Input: dimensioned drawing with shaded views. Units: mm. Origin: part minimum x, y, z. Give positions to 0.01 mm unless a question says otherwise; leave off trailing zeros. Write each loop counter-clockwise with the first axis right and the second up, starting at its lowest first coordinate (ties: lowest second). Pieces come first, ordered by that corner, then holes.
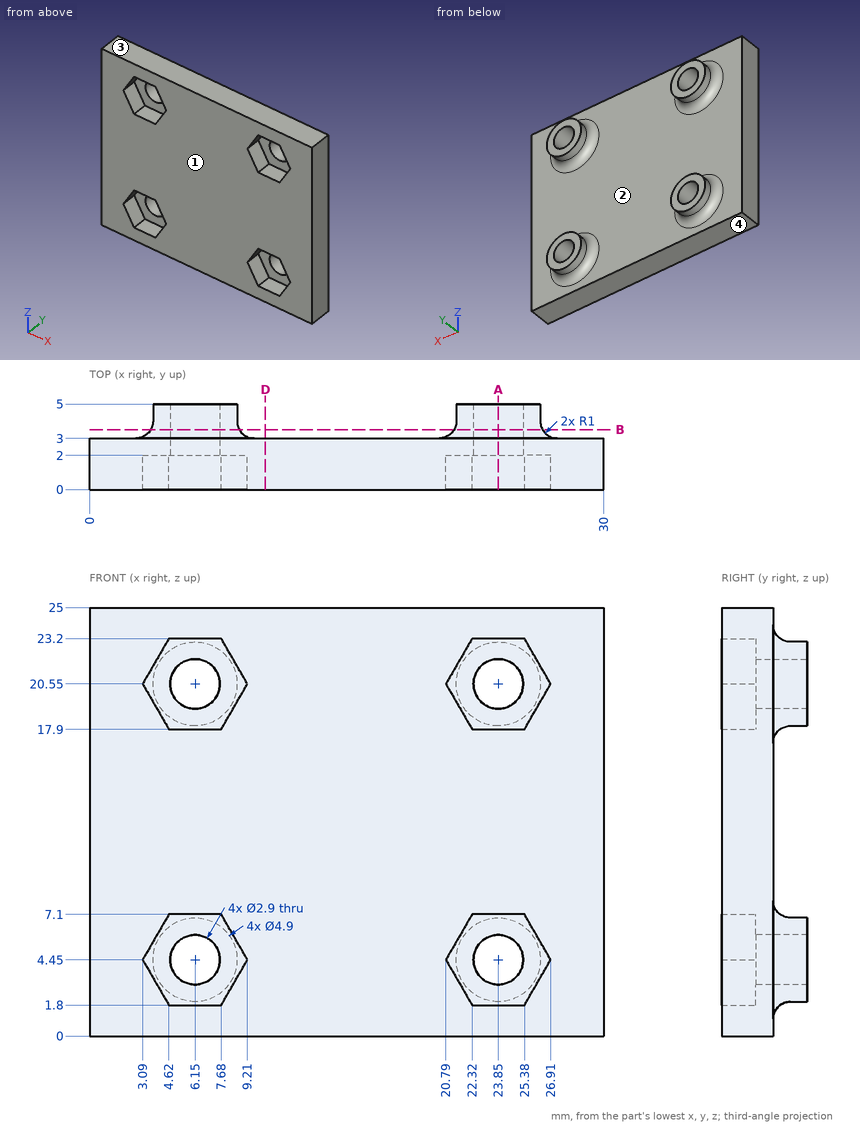
Item 1: Section B-B (y = 3.5). Return loops of the section in (x, z), and give its area (3 significant figures).
Item 2: Mould query, pull axis Z, two halves, no side actions, for the marked faces 1, 2, 3 and 4. Classes: +Z half, -Z half, draft (parallel to the pull), parting line (faces both ways), or undercut.
Item 3: Section D-D (x = 10.25). Return loops of the section in (y, z), and give its area (3 significant figures).
Item 4: Ray query, line 1 (Z direction, x = 6, y = 1.55); line 2 (Z direction, x = 6.15, y = 2.6); line 3 (X direction, y = 3.55, z = 4.45). Return the intervals inside material, ascending.
Item 5: Pin query (flat end, axial travel): pin 1 (1.6 mm diameter, centred on x = 23, z = 21.5, fed in from -Y); pin 2 (12 mm diameter, centred on x = 15, z = 5.5, fed in from +Y). Return the tip coordinate at first contact, or that it passes through.
Item 6: Section A-A (x = 23.85). Give the number of separate pieces and of enclosed holes in the cut face, and give its area (3 significant figures).
Solved:
1. outline: circle Ø5.17 at (6.15, 4.45); circle Ø5.17 at (6.15, 20.55); circle Ø5.17 at (23.85, 4.45); circle Ø5.17 at (23.85, 20.55); hole circle Ø2.9 at (6.15, 4.45); hole circle Ø2.9 at (6.15, 20.55); hole circle Ø2.9 at (23.85, 4.45); hole circle Ø2.9 at (23.85, 20.55)
1. area: 57.5 mm2
2. face 1: draft
2. face 2: undercut
2. face 3: +Z half
2. face 4: -Z half
3. outline: (0, 0) - (3, 0) - (3, 25) - (0, 25) - close
3. area: 75.0 mm2
4. line 1: z = 0 to 1.8, 7.1 to 17.9, 23.2 to 25
4. line 2: z = 0 to 3, 5.9 to 19.1, 22 to 25
4. line 3: x = 3.59 to 4.7, 7.6 to 8.71, 21.29 to 22.4, 25.3 to 26.41
5. pin 1: stops at y = 2
5. pin 2: stops at y = 3.16
6. separate pieces: 3
6. enclosed holes: 0
6. area: 56.9 mm2
